```python
from build123d import *

# Parameters (mm, degrees)
SKETCH1_R           = 30.48
SKETCH1_R_2         = 1.143
BOSS_EXTRUDE1_DEPTH = 5.08
CUT_EXTRUDE1_DEPTH  = 2.54
SKETCH3_W           = 3.556
SKETCH3_H           = 1.778
SKETCH6_R           = 26.67
SKETCH6_R_2         = 5.08
CUT_EXTRUDE2_DEPTH  = 0.508
SKETCH8_R           = 26.67
SKETCH8_R_2         = 5.08
CUT_EXTRUDE3_DEPTH  = 0.508


with BuildPart() as part:
    # Sketch1 → Boss-Extrude1 (new body)
    with BuildSketch(Plane.XY):
        Circle(SKETCH1_R)
        Circle(SKETCH1_R_2, mode=Mode.SUBTRACT)
        with BuildLine():
            Line((-1.27, 23.82731206), (-1.27, 6.599113577))
            ThreePointArc((-1.27, 6.599113577), (-1.610295474, 5.329113577), (-2.54, 4.399409051))
            ThreePointArc((-2.54, 4.399409051), (-4.399409051, 2.54), (-5.08, 0))
            ThreePointArc((-5.08, 0), (-5.420295474, -1.27), (-6.35, -2.199704526))
            Line((-6.35, -2.199704526), (-21.270057548, -10.813803767))
            ThreePointArc((-21.270057548, -10.813803767), (-23.389696909, -11.007781124), (-24.912695184, -9.52084653))
            ThreePointArc((-24.912695184, -9.52084653), (-23.096897519, 13.335), (-4.211052632, 26.335450171))
            ThreePointArc((-4.211052632, 26.335450171), (-2.161830361, 25.759962272), (-1.27, 23.82731206))
        make_face(mode=Mode.SUBTRACT)
        with BuildLine():
            Line((1.27, 23.82731206), (1.27, 6.599113577))
            ThreePointArc((1.27, 6.599113577), (1.610295474, 5.329113577), (2.54, 4.399409051))
            ThreePointArc((2.54, 4.399409051), (4.399409051, 2.54), (5.08, 0))
            ThreePointArc((5.08, 0), (5.420295474, -1.27), (6.35, -2.199704526))
            Line((6.35, -2.199704526), (21.270057548, -10.813803767))
            ThreePointArc((21.270057548, -10.813803767), (23.389696909, -11.007781124), (24.912695184, -9.52084653))
            ThreePointArc((24.912695184, -9.52084653), (23.096897519, 13.335), (4.211052632, 26.335450171))
            ThreePointArc((4.211052632, 26.335450171), (2.161830361, 25.759962272), (1.27, 23.82731206))
        make_face(mode=Mode.SUBTRACT)
        with BuildLine():
            Line((20.000057548, -13.013508293), (5.08, -4.399409051))
            ThreePointArc((5.08, -4.399409051), (3.81, -4.059113577), (2.54, -4.399409051))
            ThreePointArc((2.54, -4.399409051), (0, -5.08), (-2.54, -4.399409051))
            ThreePointArc((-2.54, -4.399409051), (-3.81, -4.059113577), (-5.08, -4.399409051))
            Line((-5.08, -4.399409051), (-20.000057548, -13.013508293))
            ThreePointArc((-20.000057548, -13.013508293), (-21.227866547, -14.752181148), (-20.701642553, -16.814603641))
            ThreePointArc((-20.701642553, -16.814603641), (0, -26.67), (20.701642553, -16.814603641))
            ThreePointArc((20.701642553, -16.814603641), (21.227866547, -14.752181148), (20.000057548, -13.013508293))
        make_face(mode=Mode.SUBTRACT)
    extrude(amount=BOSS_EXTRUDE1_DEPTH)

    # Sketch2 → Cut-Extrude1 (cut)
    with BuildSketch(Plane.XY.offset(5.08)):
        Polygon((1.770622484, 3.126255324), (-1.822105287, 3.096531714), (-3.592727772, -0.02972361), (-1.770622484, -3.126255324), (1.822105287, -3.096531714), (3.592727772, 0.02972361), align=None)
    extrude(amount=-CUT_EXTRUDE1_DEPTH, mode=Mode.SUBTRACT)

    # Sketch3 → Cut-Revolve1 (revolve, cut)
    with BuildSketch(Plane(origin=(0, 0, 0), x_dir=(0, 0, -1), z_dir=(1, 0, 0))):
        with Locations((-2.54, 29.591)):
            Rectangle(SKETCH3_W, SKETCH3_H)
    revolve(axis=Axis((0, 0, 7.917922269), (0, 0, -1)), mode=Mode.SUBTRACT)

    # Sketch6 → Cut-Extrude2 (cut)
    with BuildSketch(Plane.XY):
        Circle(SKETCH6_R)
        Circle(SKETCH6_R_2, mode=Mode.SUBTRACT)
    extrude(amount=CUT_EXTRUDE2_DEPTH, mode=Mode.SUBTRACT)

    # Sketch8 → Cut-Extrude3 (cut)
    with BuildSketch(Plane.XY.offset(5.08)):
        Circle(SKETCH8_R)
        Circle(SKETCH8_R_2, mode=Mode.SUBTRACT)
    extrude(amount=-CUT_EXTRUDE3_DEPTH, mode=Mode.SUBTRACT)


solid = part.part
```
Source: CAD feature listing. Evaluate the final solid. Frame: model axes, mm. A direction names the side the tool comes from. Round coordinates to 2 decimals unless told otherwise and drop trailing zeros. Write each loop counter-clockwise with the first axis right and the second up, starting at its lowest first coordinate (ties: lowest second). Pieces come first, ordered by that corner, then holes. Notation, with made-up numbers: M 4.25,35 L 56.25,35 A18 cw 56.25,63 Z; hole C -1.75,71 d5. An arc over 180 degrees is marked long. Use CSV: the item, a comma, the result in double quotes. Start each with the question number.
Q1. Access query for faces 1 (the face through (2.69, 1.56, 3.83)), 2 (the face through (-14, -8, 0.508)), 3 (the face through (-21.22, -14.72, 2.51)). Directions: +Z, -Z, +X, -X, +Y, -Y. A direction counts if a zero-diameter tool reaches every point of the face in a straight line with its end or side. Return the directions, or none.
Q2. First-contact query: P1, Ø8.5, axis at x = 18, y = -12, coming from the -Z side; P2, Ø1.5, axis at y = 7, z = 2, coming from the -X side; P3, Ø1.2, axis at y = 15.5, z = 2, coming from the +X side. Flat tips, straight axial feed; report the tip coordinate or a pass-through.
Q3. Pull-direction query (Z, two-part tool) for faces 4 (the face through (-2.185, 25.78, 2.512)), 5 (the face through (-27, -11, 4.318)), 6 (the face through (-0.1, -3.3, 5.08)); classes: +Z half, -Z half, draft (parallel to the pull), parting line (faces both ways), or undercut.
Q4. Cut plane D-D on x = -23. Output: boundary loops of the cut face in (y, z).
Q5. Cut plane C-C on y = -22.5. Output: boundary loops of the cut face in (x, z).
Q6. Cut plane B-B on y = 13. Output: boundary loops of the cut face in (x, z).
Q7. Line query: line 1 (X direction, y = -8.5, z = 3.7); line 2 (Y direction, x = 3, z = 0.4); line 3 (Y direction, x = 1.5, z = 2.5). Output: solid intervals per line, ascending. Write a range as from..to.
Q8. Cut plane A-A on x = -15. Output: boundary loops of the cut face in (y, z), plus the area to 3 significant figures.
Results found:
1,face 1,"+Z"
1,face 2,"-Z"
1,face 3,"+Z, -Z"
2,P1,"z = 0.51"
2,P2,"x = -28.01"
2,P3,"x = 24.53"
3,face 4,"draft"
3,face 5,"undercut"
3,face 6,"+Z half"
4,outline,"M -20,0 L -13.5,0 L -13.5,0.51 L -11.11,0.51 L -11.11,4.57 L -13.5,4.57 L -13.5,5.08 L -20,5.08 L -20,4.32 L -17.17,4.32 L -17.17,0.76 L -20,0.76 Z; M 13.5,0 L 20,0 L 20,0.76 L 17.17,0.76 L 17.17,4.32 L 20,4.32 L 20,5.08 L 13.5,5.08 Z"
5,outline,"M -20.56,0 L -14.32,0 L -14.32,5.08 L -20.56,5.08 L -20.56,4.32 L -17.82,4.32 L -17.82,0.76 L -20.56,0.76 Z; M 14.32,0 L 20.56,0 L 20.56,0.76 L 17.82,0.76 L 17.82,4.32 L 20.56,4.32 L 20.56,5.08 L 14.32,5.08 Z"
6,outline,"M -27.57,0 L -23.29,0 L -23.29,5.08 L -27.57,5.08 L -27.57,4.32 L -25.59,4.32 L -25.59,0.76 L -27.57,0.76 Z; M -1.27,0.51 L 1.27,0.51 L 1.27,4.57 L -1.27,4.57 Z; M 23.29,0 L 27.57,0 L 27.57,0.76 L 25.59,0.76 L 25.59,4.32 L 27.57,4.32 L 27.57,5.08 L 23.29,5.08 Z"
7,line 1,"-27.41..-25.28, -17.26..-12.18, 12.18..17.26, 25.28..27.41"
7,line 2,"-30.33..-26.5, -4.1..4.1, 26.5..30.33"
7,line 3,"-28.66..-26.63, -4.85..5.54, 24.88..28.66"
8,outline,"M -26.53,0 L -22.05,0 L -22.05,5.08 L -26.53,5.08 L -26.53,4.32 L -24.47,4.32 L -24.47,0.76 L -26.53,0.76 Z; M -10.13,0.51 L -7.19,0.51 L -7.19,4.57 L -10.13,4.57 Z; M 22.05,0 L 26.53,0 L 26.53,0.76 L 24.47,0.76 L 24.47,4.32 L 26.53,4.32 L 26.53,5.08 L 22.05,5.08 Z"
8,area,"42.8 mm^2"
